Autodesk Inventor part; units mm, degrees
ref_plane "YZ Plane" through (0, 0, 0) normal (1, 0, 0) x (0, 1, 0)
ref_plane "XZ Plane" through (0, 0, 0) normal (0, 1, 0) x (-1, 0, 0)
ref_plane "XY Plane" through (0, 0, 0) normal (0, 0, 1) x (1, 0, 0)
sketch "Sketch1" plane through (0, 0, 0) normal (0, 1, 0) x (-1, 0, 0)
  line L0 (-25.75, 13.25) -> (-25.75, -13.25)
  line L1 (-24.75, -14.25) -> (24.75, -14.25)
  line L2 (25.75, -13.25) -> (25.75, 13.25)
  line L3 (24.75, 14.25) -> (-24.75, 14.25)
  arc A0 (-25.75, -13.25) -> (-24.75, -14.25) centre (-24.75, -13.25) ccw
  arc A1 (-24.75, 14.25) -> (-25.75, 13.25) centre (-24.75, 13.25) ccw
  arc A2 (25.75, 13.25) -> (24.75, 14.25) centre (24.75, 13.25) ccw
  arc A3 (24.75, -14.25) -> (25.75, -13.25) centre (24.75, -13.25) ccw
  line L4 (24.75, -16.25) -> (-24.75, -16.25)
  arc A4 (-27.75, -13.25) -> (-24.75, -16.25) centre (-24.75, -13.25) ccw
  line L5 (-27.75, -13.25) -> (-27.75, 13.25)
  arc A5 (-24.75, 16.25) -> (-27.75, 13.25) centre (-24.75, 13.25) ccw
  line L6 (-24.75, 16.25) -> (24.75, 16.25)
  arc A6 (27.75, 13.25) -> (24.75, 16.25) centre (24.75, 13.25) ccw
  line L7 (27.75, 13.25) -> (27.75, -13.25)
  arc A7 (24.75, -16.25) -> (27.75, -13.25) centre (24.75, -13.25) ccw
  line L8 (21.75, -16.25) -> (21.75, -14.25)
  line L9 (27.75, -10.25) -> (25.75, -10.25)
  line L10 (25.75, 10.25) -> (27.75, 10.25)
  line L11 (21.75, 14.25) -> (21.75, 16.25)
  line L12 (-21.75, 14.25) -> (-21.75, 16.25)
  line L13 (-25.75, 10.25) -> (-27.75, 10.25)
  line L14 (-25.75, -10.25) -> (-27.75, -10.25)
  line L15 (-21.75, -16.25) -> (-21.75, -14.25)
  line L16 (-21.75, -14.25) -> (-17.75, -14.25)
  arc A8 (-17.75, -14.25) -> (-21.75, -16.25) centre (-15.3911, -23.9678) ccw
  line L17 (-21.75, 14.25) -> (-17.75, 14.25)
  arc A9 (-21.75, 16.25) -> (-17.75, 14.25) centre (-15.3911, 23.9678) ccw
  line L18 (-25.75, -10.25) -> (-25.75, -6.2495)
  line L19 (-25.75, 10.25) -> (-25.75, 6.25)
  arc A10 (-27.75, -10.25) -> (-25.75, -6.2495) centre (-35.468, -3.8913) ccw
  arc A11 (-25.75, 6.25) -> (-27.75, 10.25) centre (-35.4678, 3.8911) ccw
  line L20 (25.75, -10.25) -> (25.75, -6.2495)
  arc A12 (25.75, -6.2495) -> (27.75, -10.25) centre (35.468, -3.8913) ccw
  line L21 (25.75, 10.25) -> (25.75, 6.25)
  arc A13 (27.75, 10.25) -> (25.75, 6.25) centre (35.4678, 3.8911) ccw
  point P0 (0, 0)
  point P1 (-25.75, 14.25)
  point P2 (-25.75, -14.25)
  point P3 (25.75, -14.25)
  point P4 (21.75, 15.25)
  point P5 (-26.75, 10.25)
  dimension "d0" = 28.5
  dimension "d1" = 51.5
  dimension "d2" = 14.25
  dimension "d3" = 25.75
  dimension "d4" = 1
  dimension "d5" = 2
  dimension "d6" = 3
  dimension "d7" = 3
  dimension "d8" = 3
  dimension "d9" = 3
  dimension "d10" = 3
  dimension "d11" = 3
  dimension "d12" = 3
  dimension "d13" = 3
  dimension "d19" = 4
  dimension "d20" = 10
  dimension "d21" = 10
  dimension "d22" = 4
  dimension "d23" = 10
  dimension "d24" = 10
  dimension "d25" = 10
  dimension "d26" = 10
extrude "Extrusion1" add sketch "Sketch1" along normal blind 3.0001 contours L0 L13 L5 A5 L6 L12 L3 A1 | L0 A11 L13 | L12 A9 L3 | L0 L14 A10 | L14 L0 A0 L1 L15 L4 A4 L5 | L11 L6 A6 L7 L10 L2 A2 L3 | L15 L1 A8 | L8 L1 A3 L2 L9 L7 A7 L4 | L10 A13 L2 | L9 L2 A12
sketch "Sketch2" plane through (0, 0, 0) normal (0, -1, 0) x (1, 0, 0)
  line L0 (24.75, 14.25) -> (-24.75, 14.25)
  arc A0 (25.75, 13.25) -> (24.75, 14.25) centre (24.75, 13.25) ccw
  line L1 (-24.75, 14.25) -> (24.75, 14.25)
  line L2 (25.75, -13.25) -> (25.75, 13.25)
  line L3 (-24.75, -14.25) -> (24.75, -14.25)
  arc A1 (-25.75, -13.25) -> (-24.75, -14.25) centre (-24.75, -13.25) ccw
  arc A2 (24.75, -14.25) -> (25.75, -13.25) centre (24.75, -13.25) ccw
  line L4 (-25.75, 13.25) -> (-25.75, -13.25)
  arc A3 (-24.75, 14.25) -> (-25.75, 13.25) centre (-24.75, 13.25) ccw
  line L5 (24.75, -16.25) -> (-24.75, -16.25)
  arc A4 (-27.75, -13.25) -> (-24.75, -16.25) centre (-24.75, -13.25) ccw
  line L6 (-27.75, -13.25) -> (-27.75, 13.25)
  arc A5 (-24.75, 16.25) -> (-27.75, 13.25) centre (-24.75, 13.25) ccw
  line L7 (-24.75, 16.25) -> (24.75, 16.25)
  arc A6 (27.75, 13.25) -> (24.75, 16.25) centre (24.75, 13.25) ccw
  line L8 (27.75, 13.25) -> (27.75, -13.25)
  arc A7 (24.75, -16.25) -> (27.75, -13.25) centre (24.75, -13.25) ccw
  point P0 (0, 0)
  dimension "d16" = 2
extrude "Extrusion2" add sketch "Sketch2" against normal blind 3 contours A0 L2 A2 L3 A1 L4 A3 L0
sketch "Sketch3" plane through (0, 3, 0) normal (0, 1, 0) x (1, 0, 0)
  line L0 (6.7, 10.65) -> (24.9, 10.65)
  line L1 (24.9, 10.65) -> (24.9, -10.65)
  line L2 (24.9, -10.65) -> (6.7, -10.65)
  line L3 (6.7, -10.65) -> (6.7, 10.65)
  line L4 (-5.6, 11.1) -> (5.6, 11.1)
  line L5 (5.6, 11.1) -> (5.6, -11.1)
  line L6 (5.6, -11.1) -> (-5.6, -11.1)
  line L7 (-5.6, -11.1) -> (-5.6, 11.1)
  line L8 (17.75, 14.25) -> (-21.75, 14.25)
  line L9 (-21.75, -14.25) -> (17.75, -14.25)
  line L10 (-6.7, -10.65) -> (-24.9, -10.65)
  line L11 (-6.7, 10.65) -> (-6.7, -10.65)
  line L12 (-24.9, 10.65) -> (-6.7, 10.65)
  line L13 (-24.9, -10.65) -> (-24.9, 10.65)
  point P0 (0, 0)
  dimension "d27" = 18.2
  dimension "d28" = 21.3
  dimension "d29" = 10.65
  dimension "d30" = 6.7
  dimension "d31" = 11.2
  dimension "d32" = 22.2
  dimension "d33" = 5.6
  dimension "d34" = 11.1
  dimension "d69" = 360
extrude "Extrusion3" cut sketch "Sketch3" against normal blind 2
sketch "Sketch4" plane through (0, 3, 0) normal (0, 1, 0) x (1, 0, 0)
  line L0 (-25.75, 6.2495) -> (-25.75, 13.25)
  line L1 (-25.75, 12.05) -> (-23.55, 12.05)
  line L2 (-24.75, 14.25) -> (-21.75, 14.25)
  line L3 (-23.55, 14.25) -> (-23.55, 12.05)
  circle A0 centre (-23.55, 12.05) radius 1.4
  line L4 (17.75, 14.25) -> (24.75, 14.25)
  line L5 (23.55, 14.25) -> (23.55, 12.05)
  line L6 (25.75, 13.25) -> (25.75, 6.2495)
  line L7 (25.75, 12.05) -> (23.55, 12.05)
  line L8 (24.75, -14.25) -> (17.75, -14.25)
  line L9 (23.55, -14.25) -> (23.55, -12.05)
  line L10 (25.75, -6.25) -> (25.75, -13.25)
  line L11 (25.75, -12.05) -> (23.55, -12.05)
  line L12 (-25.75, -13.25) -> (-25.75, -6.25)
  line L13 (-25.75, -12.05) -> (-23.55, -12.05)
  line L14 (-21.75, -14.25) -> (-24.75, -14.25)
  line L15 (-23.55, -14.25) -> (-23.55, -12.05)
  point P0 (0, 0)
  dimension "d39" = 2.2
  dimension "d40" = 2.2
  dimension "d41" = 2.8
  dimension "d42" = 2.2
  dimension "d43" = 2.2
  dimension "d44" = 2.2
  dimension "d45" = 2.2
  dimension "d46" = 2.2
  dimension "d48" = 2.2
hole "Hole1" at (-23.55, 3, -12.05) at (23.55, 3, -12.05) at (23.55, 3, 12.05) at (-23.55, 3, 12.05) direction (0, -1, 0) diameter 2.8 end through all
sketch "Sketch5" plane through (0, 0, 0) normal (0, -1, 0) x (1, 0, 0)
  line L0 (25.75, -13.25) -> (25.75, -6.2495)
  arc A0 (25.75, -6.2495) -> (27.75, -10.25) centre (35.468, -3.8913) ccw
  line L1 (27.75, -10.25) -> (27.75, -13.25)
  arc A1 (24.75, -16.25) -> (27.75, -13.25) centre (24.75, -13.25) ccw
  line L2 (24.75, -16.25) -> (21.75, -16.25)
  arc A2 (21.75, -16.25) -> (17.75, -14.25) centre (15.3911, -23.9678) ccw
  line L3 (17.75, -14.25) -> (24.75, -14.25)
  arc A3 (24.75, -14.25) -> (25.75, -13.25) centre (24.75, -13.25) ccw
  line L4 (25.75, 6.25) -> (25.75, 13.25)
  arc A4 (27.75, 10.25) -> (25.75, 6.25) centre (35.4678, 3.8911) ccw
  line L5 (27.75, 13.25) -> (27.75, 10.25)
  arc A5 (27.75, 13.25) -> (24.75, 16.25) centre (24.75, 13.25) ccw
  arc A6 (25.75, 13.25) -> (24.75, 14.25) centre (24.75, 13.25) ccw
  line L6 (24.75, 14.25) -> (17.75, 14.25)
  arc A7 (17.75, 14.25) -> (21.75, 16.25) centre (15.3911, 23.9678) ccw
  line L7 (21.75, 16.25) -> (24.75, 16.25)
  line L8 (-21.75, 14.25) -> (-24.75, 14.25)
  line L9 (-21.75, 16.25) -> (-21.75, 14.25)
  line L10 (-24.75, 16.25) -> (-21.75, 16.25)
  arc A8 (-24.75, 16.25) -> (-27.75, 13.25) centre (-24.75, 13.25) ccw
  line L11 (-27.75, 10.25) -> (-27.75, 13.25)
  arc A9 (-25.75, 6.25) -> (-27.75, 10.25) centre (-35.4678, 3.8911) ccw
  line L12 (-25.75, 13.25) -> (-25.75, 6.25)
  arc A10 (-24.75, 14.25) -> (-25.75, 13.25) centre (-24.75, 13.25) ccw
  line L13 (-27.75, -13.25) -> (-27.75, -10.25)
  arc A11 (-27.75, -13.25) -> (-24.75, -16.25) centre (-24.75, -13.25) ccw
  line L14 (-21.75, -16.25) -> (-24.75, -16.25)
  line L15 (-21.75, -14.25) -> (-21.75, -16.25)
  line L16 (-24.75, -14.25) -> (-21.75, -14.25)
  arc A12 (-25.75, -13.25) -> (-24.75, -14.25) centre (-24.75, -13.25) ccw
  line L17 (-25.75, -6.2495) -> (-25.75, -13.25)
  arc A13 (-27.75, -10.25) -> (-25.75, -6.2495) centre (-35.468, -3.8913) ccw
  point P0 (0, 0)
extrude "Extrusion4" add sketch "Sketch5" along normal blind 9
sketch "Sketch6" plane through (0, 3, 0) normal (0, 1, 0) x (1, 0, 0)
  line L0 (17.75, 14.25) -> (-21.75, 14.25)
  arc A0 (-6.1051, 14.25) -> (-8, 17.039) centre (-9.1051, 14.25) ccw
  line L1 (-8, 17.039) -> (-8, 18.039)
  line L2 (-8, 18.039) -> (8, 18.039)
  line L3 (8, 18.039) -> (8, 17.039)
  arc A1 (8, 17.039) -> (5.6575, 14.25) centre (8.6543, 14.1113) ccw
  line L4 (-5.6, 11.1) -> (5.6, 11.1)
  line L5 (-24.5, 0) -> (24.9, 0)
  line L6 (24.9, 10.65) -> (24.9, -10.65)
  arc A2 (-8, -17.039) -> (-6.1051, -14.25) centre (-9.1051, -14.25) ccw
  line L7 (-8, -17.039) -> (-8, -18.039)
  line L8 (-8, -18.039) -> (8, -18.039)
  line L9 (8, -18.039) -> (8, -17.039)
  arc A3 (5.6575, -14.25) -> (8, -17.039) centre (8.6543, -14.1113) ccw
  line L10 (-6.1051, -14.25) -> (5.6575, -14.25)
  line L11 (-6.1051, 14.25) -> (5.6575, 14.25)
  point P0 (0, 0)
  point P1 (0, 11.1)
  dimension "d58" = 3
  dimension "d59" = 1
  dimension "d60" = 1
  dimension "d61" = 3
  dimension "d62" = 16
  dimension "d63" = 8
extrude "Extrusion5" add sketch "Sketch6" against normal blind 3
sketch "Sketch7" plane through (0, 1, 0) normal (0, 1, 0) x (1, 0, 0)
  line L0 (-24.9, -10.65) -> (-24.9, 10.65)
  line L1 (-24.9, 10.65) -> (-21.9, 10.65)
  line L2 (-23.55, 10.65) -> (-6.7, 10.65)
  line L3 (-21.9, 10.65) -> (-21.9, -10.65)
  line L4 (-6.7, -10.65) -> (-23.55, -10.65)
  line L5 (-21.9, -10.65) -> (-24.9, -10.65)
  line L6 (-24.9, 10.65) -> (-24.9, -10.65)
  line L7 (-6.7, 10.65) -> (-6.7, -10.65)
  line L8 (-6.7, 10.65) -> (-9.7, 10.65)
  line L9 (-9.7, 10.65) -> (-9.7, -10.65)
  line L10 (-9.7, -10.65) -> (-6.7, -10.65)
  line L11 (-6.7, 10.65) -> (-6.7, -10.65)
  line L12 (-5.6, 11.1) -> (5.6, 11.1)
  line L13 (-5.6, 11.1) -> (-5.6, 7.6)
  line L14 (-5.6, 7.6) -> (5.6, 7.6)
  line L15 (5.6, 7.6) -> (5.6, 11.1)
  line L16 (5.6, 11.1) -> (-5.6, 11.1)
  line L17 (5.6, -11.1) -> (-5.6, -11.1)
  line L18 (-5.6, -11.1) -> (-5.6, -7.6)
  line L19 (-5.6, -11.1) -> (-5.6, 11.1)
  line L20 (-5.6, -7.6) -> (6.15, -7.6)
  line L21 (6.15, -7.6) -> (6.15, -11.1)
  line L22 (6.15, -11.1) -> (-5.6, -11.1)
  line L23 (6.7, 10.65) -> (23.55, 10.65)
  line L24 (6.7, 10.65) -> (9.7, 10.65)
  line L25 (9.7, 10.65) -> (9.7, -10.65)
  line L26 (23.55, -10.65) -> (6.7, -10.65)
  line L27 (6.7, -10.65) -> (6.7, 10.65)
  line L28 (23.55, 10.65) -> (24.9, 10.65)
  line L29 (24.9, 10.65) -> (21.9, 10.65)
  line L30 (21.9, 10.65) -> (21.9, -10.65)
  line L31 (24.9, 10.65) -> (24.9, -10.65)
  line L32 (24.9, -10.65) -> (24.9, 10.65)
  line L33 (24.9, 10.65) -> (24.9, -10.65)
  line L34 (21.9, -10.65) -> (24.9, -10.65)
  line L35 (21.9, 10.65) -> (24.9, 10.65)
  point P0 (0, 0)
  point P1 (5.875, -11.3)
  point P2 (-23.55, -10.65)
  dimension "d71" = 3
  dimension "d72" = 3
  dimension "d73" = 3.5
  dimension "d74" = 3.5
  dimension "d75" = 3
  dimension "d76" = 3
extrude "Extrusion6" cut sketch "Sketch7" against normal through all contours L0 L1 L3 L4 L5 | L9 L2 L7 L4 | L20 L21 L22 L17 L18 | L12 L15 L14 L13 | L23 L25 L26 L27 | L23 L28 L31 L34 L26 L30
sketch "Sketch9" plane through (0, 3.0001, 0) normal (0, 1, 0) x (1, 0, 0)
  line L0 (-24.9, 10.65) -> (-23.55, 10.65)
  line L1 (-24.9, 10.65) -> (-25.75, 10.65)
  line L2 (-25.75, 6.2495) -> (-25.75, 13.25)
  line L3 (-27.75, 13.25) -> (-27.75, 10.25)
  arc A0 (-25.75, 10.65) -> (-27.75, 13.25) centre (-28.1706, 10.8572) ccw
  line L4 (-25.75, 10.65) -> (-25.75, -10.65)
  line L5 (-25.75, -13.25) -> (-25.75, -6.25)
  line L6 (-25.75, -10.65) -> (25.7428, -10.65)
  line L7 (23.55, -10.65) -> (6.7, -10.65)
  line L8 (25.75, 13.25) -> (25.75, 6.2495)
  line L9 (25.75, 10.65) -> (-25.75, 10.65)
  arc A1 (27.75, 13.25) -> (24.75, 16.25) centre (24.75, 13.25) ccw
  arc A2 (27.75, 13.25) -> (25.75, 10.65) centre (28.4412, 10.6491) ccw
  arc A3 (24.75, -16.25) -> (27.75, -13.25) centre (24.75, -13.25) ccw
  arc A4 (25.7428, -10.65) -> (27.75, -13.25) centre (28.4291, -10.6509) ccw
  line L10 (24.75, -14.25) -> (17.75, -14.25)
  line L11 (-27.75, -10.25) -> (-27.75, -13.25)
  arc A5 (-27.75, -13.25) -> (-25.75, -10.65) centre (-28.44, -10.65) ccw
  arc A6 (-25.75, 6.2495) -> (-27.75, 10.25) centre (-35.468, 3.8913) ccw
  arc A7 (-27.75, -10.25) -> (-25.75, -6.25) centre (-35.4678, -3.8911) ccw
  arc A8 (21.75, -16.25) -> (17.75, -14.25) centre (15.3911, -23.9678) ccw
  line L12 (21.75, -16.25) -> (24.75, -16.25)
  line L13 (27.75, -13.25) -> (27.75, -10.25)
  arc A9 (25.75, -6.25) -> (27.75, -10.25) centre (35.4678, -3.8911) ccw
  line L14 (25.75, -6.25) -> (25.75, -13.25)
  line L15 (25.75, 13.25) -> (25.75, 6.2495)
  arc A10 (27.75, 10.25) -> (25.75, 6.2495) centre (35.468, 3.8913) ccw
  line L16 (27.75, 10.25) -> (27.75, 13.25)
  line L17 (24.75, 16.25) -> (21.75, 16.25)
  arc A11 (17.75, 14.25) -> (21.75, 16.25) centre (15.3911, 23.9678) ccw
  line L18 (17.75, 14.25) -> (24.75, 14.25)
  line L19 (21.75, 16.25) -> (21.75, 14.25)
  line L20 (21.75, -16.25) -> (21.75, -14.25)
  point P0 (0, 0)
  point P1 (25.75, -10.848)
  point P2 (-25.75, 11.0644)
  dimension "d84" = 2.4295
  dimension "d86" = 0
extrude "Extrusion8" cut sketch "Sketch9" against normal through all contours L19 L18 A11 | A2 L16 A10 L8 | A8 L10 L20 | L14 A9 L13 A4 | L4 A5 L11 A7 | L2 A6 L3 A0
Geometry: final body of the model. Coordinates: model frame, mm. A direction names the side the tool comes from. Give positions to 0.01 mm unless a question says otherwise; leave off trailing zeros. Write each loop counter-clockwise with the first axis right and the second up, starting at its lowest first coordinate (ties: lowest second). Pieces come first, ordered by that corner, then holes. Notation, with made-up numbers: M -27,49.25 L 2,49.25 A12 ccw 2,65.25 Z; hole C -37.75,-36.5 d6. An arc over 180 degrees is marked long. Answer in a Markdown table with one row per item. Add a question column.
(1) Mould query, pull axis Z, two halves, no side actions, for faces 1 (the flat face through (25, -9, -15)), 2 (the flat face through (0, 2, -18.039)), 3 (the cylindrical face through (26.323, -2.916, -12.309)). Classes: +Z half, -Z half, draft (parallel to the pull), parting line (faces both ways), or undercut.
(2) Ray query, line 1 (Z direction, x = -4, y = 0.25); line 2 (X direction, y = 0.5, z = -8); line 3 (X direction, y = 1, z = -12.05). Return the intervals inside material, ascending.
(3) Section A-A on z = -9.5. Return loops of the section in (x, y), and give its area (3 significant figures).
(4) Section C-C on y = -1. Return loops of the section in (x, z), and give its area (3 significant figures).
(5) Reachability of faces 4 (the flat face through (23, -3, -16.25)), 5 (the flat face through (-16, 1, 0)), 6 (the flat face through (-21.75, -3, 15)), 7 (the cylindrical face through (-6.64, 1.52, 15.96)), 8 (the flat face through (23, -4, -14.25)) from +Z, -Z, +X, -X, +Y, -Y: full face, straight path, thin tool, end or side. Return the list, or none.
(6) Section D-D on x = -2. Return loops of the section in (y, z).
(7) First-contact query: pin 1 (1.5 mm diameter, centred on x = -3, z = 3, fed in from -Y); pin 2 (6 mm diameter, centred on x = 1, z = 6.5, fed in from +Y); pin 3 (2.5 mm diameter, centred on y = 2, z = 4.5, fed in from -X); pin 4 (5 mm diameter, centred on x = 4.5, y = -4.5, fed in from -Z). Flat tips, straight axial feed; report the tip coordinate or a pass-through.
(8) Section B-B on x = 9. Return loops of the section in (y, z), and give its area (3 significant figures).
Result set:
| question | item | result |
|---|---|---|
| 1 | face 1 | draft |
| 1 | face 2 | -Z half |
| 1 | face 3 | undercut |
| 2 | line 1 | z = -18.04 to -11.1, -7.6 to 7.6, 11.1 to 18.04 |
| 2 | line 2 | x = -25.75 to -24.9, -21.9 to -9.7, -6.7 to -5.6, 5.6 to 6.7, 9.7 to 21.9, 24.9 to 25.75 |
| 2 | line 3 | x = -26.05 to -24.95, -22.15 to 22.15, 24.95 to 26.14 |
| 3 | outline | M -25.75,0 L -24.9,0 L -24.9,3 L -25.75,3 Z; M -21.9,0 L -9.7,0 L -9.7,1 L -21.9,1 Z; M -6.7,0 L -5.6,0 L -5.6,3 L -6.7,3 Z; M 5.6,0 L 6.7,0 L 6.7,3 L 5.6,3 Z; M 9.7,0 L 21.9,0 L 21.9,1 L 9.7,1 Z; M 24.9,0 L 25.75,0 L 25.75,3 L 24.9,3 Z |
| 3 | area | 36.1 mm^2 |
| 4 | outline | M -27.75,-13.25 A3 ccw -24.75,-16.25 L -21.75,-16.25 L -21.75,-14.25 L -24.75,-14.25 A1 cw -25.75,-13.25 L -25.75,-11.06 A2.43 cw Z; M -27.75,13.25 A2.69 cw -25.75,10.65 L -25.75,13.25 A1 cw -24.75,14.25 L -21.75,14.25 L -21.75,16.25 L -24.75,16.25 A3 ccw Z; M 21.75,-16.25 L 24.75,-16.25 A3 ccw 27.75,-13.25 A2.69 cw 25.75,-10.65 L 25.75,-13.25 A1 cw 24.75,-14.25 L 21.75,-14.25 Z; M 21.75,14.25 L 24.75,14.25 A1 cw 25.75,13.25 L 25.75,10.85 A2.69 cw 27.75,13.25 A3 ccw 24.75,16.25 L 21.75,16.25 Z |
| 4 | area | 54.3 mm^2 |
| 5 | face 4 | -Z, +X, +Y, -Y |
| 5 | face 5 | +Y |
| 5 | face 6 | +Z, +Y, -Y |
| 5 | face 7 | +Y, -Y |
| 5 | face 8 | -Y |
| 6 | outline | M 0,-18.04 L 3,-18.04 L 3,-11.1 L 0,-11.1 Z; M 0,-7.6 L 1,-7.6 L 1,7.6 L 0,7.6 Z; M 0,11.1 L 3,11.1 L 3,18.04 L 0,18.04 Z |
| 7 | pin 1 | stops at y = 0 |
| 7 | pin 2 | stops at y = 1 |
| 7 | pin 3 | stops at x = -25.75 |
| 7 | pin 4 | passes through |
| 8 | outline | M 0,-14.25 L 3,-14.25 L 3,-10.65 L 0,-10.65 Z; M 0,10.65 L 3,10.65 L 3,14.25 L 0,14.25 Z |
| 8 | area | 21.6 mm^2 |
